Input: part model. Units: mm. Frame: model coordinates. Face numbers are marked on the shaded views. Give positions to 0.01 mm unless a question says otherwise; leave off trailing zeros. Loops run counter-clockwise (first coordinate to the right, second up) from the corner with the lowest first, then second, coordinate; pieces in that order, holes last. Notation, with made-up numbers: (74, 18) - (131, 18) arc R22 cw to (131, 27) - close; hole circle Ø6 at (69.5, -31). An arc over 180 degrees is marked (long way). Answer as a JSON object with one key per item and string values.
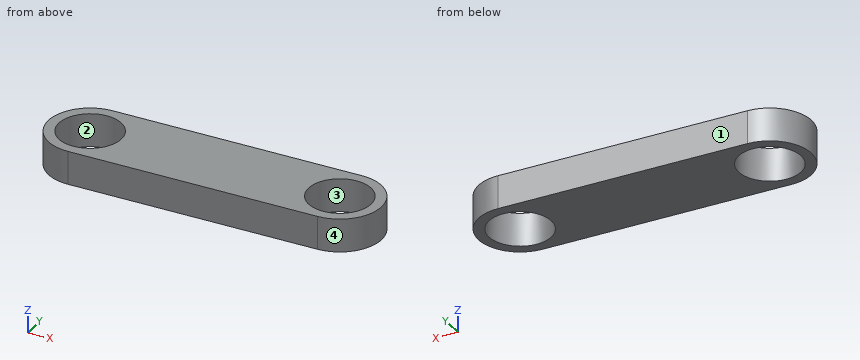
from build123d import *

# Parameters (mm, degrees)
BOSS_EXTRUDE1_DEPTH      = 40
BOSS_EXTRUDE1_DEPTH_BACK = 40
CUT_EXTRUDE1_DEPTH       = 200
CUT_EXTRUDE1_DEPTH_BACK  = 200
SKETCH7_R                = 75
CUT_EXTRUDE2_DEPTH       = 200
CUT_EXTRUDE2_DEPTH_BACK  = 200
SKETCH8_R                = 75


with BuildPart() as part:
    # Sketch2 → Boss-Extrude1 (new, two sides: drawn at the far end of the back side and taken through both)
    with BuildSketch(Plane.XY.offset(-BOSS_EXTRUDE1_DEPTH_BACK)):
        with BuildLine():
            Line((600, 100), (0, 100))
            ThreePointArc((0, 100), (-100, 0), (0, -100))
            Line((0, -100), (600, -100))
            ThreePointArc((600, -100), (700, 0), (600, 100))
        make_face()
    extrude(amount=BOSS_EXTRUDE1_DEPTH + BOSS_EXTRUDE1_DEPTH_BACK)

    # Sketch7 → Cut-Extrude1 (cut, two sides: drawn at the far end of the back side and taken through both)
    with BuildSketch(Plane.XY.offset(-CUT_EXTRUDE1_DEPTH_BACK)):
        Circle(SKETCH7_R)
    extrude(amount=CUT_EXTRUDE1_DEPTH + CUT_EXTRUDE1_DEPTH_BACK, mode=Mode.SUBTRACT)

    # Sketch8 → Cut-Extrude2 (cut, two sides: drawn at the far end of the back side and taken through both)
    with BuildSketch(Plane.XY.offset(-CUT_EXTRUDE2_DEPTH_BACK)):
        with Locations((600, 0)):
            Circle(SKETCH8_R)
    extrude(amount=CUT_EXTRUDE2_DEPTH + CUT_EXTRUDE2_DEPTH_BACK, mode=Mode.SUBTRACT)


solid = part.part
Item 1: Cut plane D-D (y = -31.5). Return loops of the section in (x, z).
Geometry check:
{"outline": "(-94.91, -40) - (-68.06, -40) - (-68.06, 40) - (-94.91, 40) - close; (68.06, -40) - (531.94, -40) - (531.94, 40) - (68.06, 40) - close; (668.06, -40) - (694.91, -40) - (694.91, 40) - (668.06, 40) - close"}
Item 2: Mould query, pull axis Y, two halves, no side actions, for the marked faces 1, 2, 3 and 4. Classes: released by +Y, released by -Y, zero draft, split by the parting line, or undercut.
Geometry check:
{"face 1": "released by +Y", "face 2": "undercut", "face 3": "undercut", "face 4": "split by the parting line"}
Item 3: Material intervals for line 1 (X direction, y = 0, z = 18); line 2 (Y direction, x = 600, z = -22); line 3 (X direction, y = 46, z = 30.5), sorted ascending. Write a range as [from, to].
Geometry check:
{"line 1": "x = [-100, -75], [75, 525], [675, 700]", "line 2": "y = [-100, -75], [75, 100]", "line 3": "x = [-88.79, -59.24], [59.24, 540.76], [659.24, 688.79]"}
Item 4: Contact query for flat-ended pins moving along their axis: P1, Ø1, axis at y = -77.5, z = 8, coming from the -X side; P2, Ø1, axis at y = -56, z = -18, coming from the -X side; P3, Ø1.5, axis at y = 53, z = -3, coming from the +X side. Output: stop coordinate, or through.
Geometry check:
{"P1": "stops at x = -63.8", "P2": "stops at x = -83.19", "P3": "stops at x = 685.26"}
Item 5: Cut plane C-C (z = -20). Return loops of the section in (x, y).
Geometry check:
{"outline": "(0, -100) - (600, -100) arc R100 ccw to (600, 100) - (0, 100) arc R100 ccw to start; hole circle Ø150 at (0, 0); hole circle Ø150 at (600, 0)"}
Item 6: Cut plane B-B (x = -42). Return loops of the section in (y, z), then the cut area to 3 significant figures.
Geometry check:
{"outline": "(-90.75, -40) - (-62.14, -40) - (-62.14, 40) - (-90.75, 40) - close; (62.14, -40) - (90.75, -40) - (90.75, 40) - (62.14, 40) - close", "area": "4,580 mm2"}
Item 7: Cut plane A-A (y = 0). Return loops of the section in (x, z), then the cut area to 3 significant figures.
Geometry check:
{"outline": "(-100, -40) - (-75, -40) - (-75, 40) - (-100, 40) - close; (75, -40) - (525, -40) - (525, 40) - (75, 40) - close; (675, -40) - (700, -40) - (700, 40) - (675, 40) - close", "area": "40,000 mm2"}
